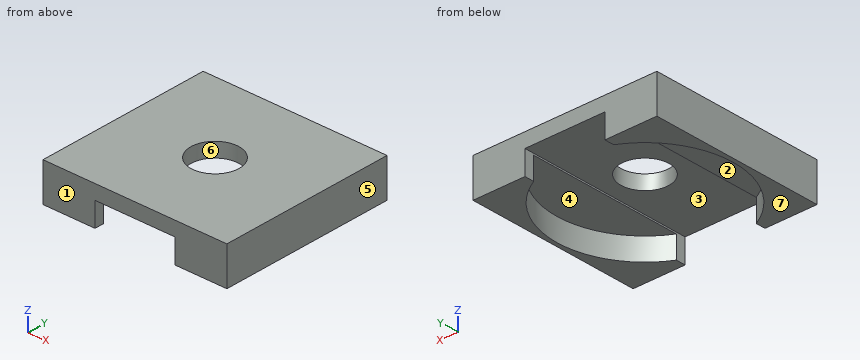
from build123d import *

# Parameters (mm, degrees)
F0_W     = 23
F0_H     = 22
F0_R     = 3
F1_DEPTH = 1.8
F3_DEPTH = 0.2
F4_DEPTH = 3


with BuildPart() as f1:
    # F0 (on Top) → F1 (new body)
    with BuildSketch(Plane.XY):
        Rectangle(F0_W, F0_H)
        Circle(F0_R, mode=Mode.SUBTRACT)
    extrude(amount=F1_DEPTH)

    # F2 (on face) → F3 (join)
    with BuildSketch(Plane(origin=(0, 0, 0), x_dir=(1, 0, 0), z_dir=(0, 0, -1))):
        with BuildLine():
            Line((-5, -9.797959), (-5, 9.797959))
            ThreePointArc((-5, 9.797959), (-11, 0), (-5, -9.797959))
        make_face()
        with BuildLine():
            ThreePointArc((5, -9.797959), (11, 0), (5, 9.797959))
            Line((5, 9.797959), (5, -9.797959))
        make_face()
    extrude(amount=F3_DEPTH)

    # F2 (on face) → F4 (join)
    with BuildSketch(Plane(origin=(0, 0, 0), x_dir=(1, 0, 0), z_dir=(0, 0, -1))):
        with BuildLine():
            Line((-5, 9.797959), (-5, 11))
            Line((-5, 11), (-11.5, 11))
            Line((-11.5, 11), (-11.5, -11))
            Line((-11.5, -11), (-5, -11))
            Line((-5, -11), (-5, -9.797959))
            ThreePointArc((-5, -9.797959), (-11, 0), (-5, 9.797959))
        make_face()
        with BuildLine():
            Line((11.5, 11), (5, 11))
            Line((5, 11), (5, 9.797959))
            ThreePointArc((5, 9.797959), (11, 0), (5, -9.797959))
            Line((5, -9.797959), (5, -11))
            Line((5, -11), (11.5, -11))
            Line((11.5, -11), (11.5, 11))
        make_face()
    extrude(amount=F4_DEPTH)


solid = f1.part
Verification items for the finished model (mm, model axes). Face numbers are marked on the shaded views. A direction names the side the tool comes from. Give positions to 0.01 mm unless a question says otherwise; leave off trailing zeros. Order: outer loops, then holes, each group sorted by start corner. A loop starts at its lowest first (then second) coordinate and runs counter-clockwise, first axis right, second up. Notation, with made-up numbers: M 66.5,17.5 L 73.5,17.5 A27 ccw 73.5,54.5 Z; hole C -18.75,53 d8. An arc over 180 degrees is marked long. Answer as a JSON object with one key per item and string values. Group by question number.
1) Depth check by flat-ended pin: pin 1 Ø3 at (x, y) = (-1.5, 5) entering from -Z; pin 2 Ø1.8 at (x, y) = (6.5, 0) entering from -Z. Enter the tip coordinate at first touch or a pass-through.
2) Scan lines: line 1 along X through (y, z) = (-4.75, -0.15); line 2 along Z through (x, y) = (0.5, -3); line 3 along X through (y, z) = (-0.25, 0.55). Record each from-to range of solid material in increasing order. Write a range as [from, to].
3) Access from +Z, -Z, +X, -X, +Y, -Y to the whole of each face (thin tool, end or side, straight path). Record for the marked faces 1, 2 and 3.
4) Cross-section at A-A (x = 0). Enter the section's corners in (y, z).
5) Cross-section at B-B (y = 0). Enter the section's corners in (x, z), then the cut area to 3 significant figures.
6) Mould release check, pull along X, two halves, no side actions. Record for the marked faces 4, 5, 6 and 7: released by +X, released by -X, zero draft, split by the parting line, or undercut.
7) Cross-section at C-C (z = -2.5). Enter the section's corners in (x, y).
8) Cross-section at D-D (z = 0.75). Enter the section's corners in (x, y).
Result sheet:
{
 "1": {"pin 1": "stops at z = 0", "pin 2": "stops at z = -0.2"},
 "2": {"line 1": "x = [-11.5, -5], [5, 11.5]", "line 2": "z = [0, 1.8]", "line 3": "x = [-11.5, -2.99], [2.99, 11.5]"},
 "3": {"face 1": "+Z, -Z, +X, -X, -Y", "face 2": "-Z", "face 3": "-Z, +Y, -Y"},
 "4": {"outline": "M -11,0 L -3,0 L -3,1.8 L -11,1.8 Z; M 3,0 L 11,0 L 11,1.8 L 3,1.8 Z"},
 "5": {"outline": "M -11.5,-3 L -11,-3 L -11,-0.2 L -5,-0.2 L -5,0 L -3,0 L -3,1.8 L -11.5,1.8 Z; M 3,0 L 5,0 L 5,-0.2 L 11,-0.2 L 11,-3 L 11.5,-3 L 11.5,1.8 L 3,1.8 Z", "area": "36.0 mm2"},
 "6": {"face 4": "undercut", "face 5": "released by +X", "face 6": "undercut", "face 7": "zero draft"},
 "7": {"outline": "M -11.5,-11 L -5,-11 L -5,-9.8 A11 cw -5,9.8 L -5,11 L -11.5,11 Z; M 5,-11 L 11.5,-11 L 11.5,11 L 5,11 L 5,9.8 A11 cw 5,-9.8 Z"},
 "8": {"outline": "M -11.5,-11 L 11.5,-11 L 11.5,11 L -11.5,11 Z; hole C 0,0 d6"}
}
